from build123d import *

# Parameters (mm, degrees)
SKETCH2_W           = 1200
SKETCH2_H           = 1200
BOSS_EXTRUDE1_DEPTH = 600
SHELL1_T            = -100
SKETCH4_W           = 1200
SKETCH4_H           = 1200
BOSS_EXTRUDE2_DEPTH = 100
SKETCH5_R           = 129.5
CUT_EXTRUDE2_DEPTH  = 601
SKETCH7_W           = 130
SKETCH7_H           = 130
CUT_EXTRUDE3_DEPTH  = 146
CIRPATTERN1_COUNT   = 4
SKETCH8_R           = 120
CUT_EXTRUDE4_DEPTH  = 100


with BuildPart() as part:
    # Sketch2 → Boss-Extrude1 (new body)
    with BuildSketch(Plane.XY):
        Rectangle(SKETCH2_W, SKETCH2_H)
    extrude(amount=BOSS_EXTRUDE1_DEPTH)

    # Shell1
    shell1_openings = [part.faces().sort_by_distance(p)[0] for p in [
        (0, 0, 600),
    ]]
    offset(amount=SHELL1_T, openings=shell1_openings, kind=Kind.INTERSECTION)

    # Sketch4 → Boss-Extrude2 (add)
    with BuildSketch(Plane.XY.offset(600)):
        Rectangle(SKETCH4_W, SKETCH4_H)
    extrude(amount=-BOSS_EXTRUDE2_DEPTH)

    # Sketch5 → Cut-Extrude2 (cut, through all)
    with BuildSketch(Plane(origin=(0, 0, 0), x_dir=(-1, 0, 0), z_dir=(0, 0, -1))):
        Circle(SKETCH5_R)
    extrude(amount=-CUT_EXTRUDE2_DEPTH, mode=Mode.SUBTRACT)

    # Sketch7 → Cut-Extrude3 (cut)
    with BuildSketch(Plane(origin=(0, 0, 0), x_dir=(-1, 0, 0), z_dir=(0, 0, -1))):
        with Locations((0, 310)):
            Rectangle(SKETCH7_W, SKETCH7_H)
    cut_extrude3 = extrude(amount=-CUT_EXTRUDE3_DEPTH, mode=Mode.SUBTRACT)

    # CirPattern1: Cut-Extrude3 ×4 about axis
    cirpattern1_axis = Axis((0, 0, 0), (0, 0, 1))
    for i in range(1, CIRPATTERN1_COUNT):
        add(cut_extrude3.rotate(cirpattern1_axis, i * 360 / CIRPATTERN1_COUNT), mode=Mode.SUBTRACT)

    # Sketch8 → Cut-Extrude4 (cut)
    with BuildSketch(Plane.XZ.offset(600)):
        with Locations((-344.367385343, 324.291039311)):
            Circle(SKETCH8_R)
    extrude(amount=-CUT_EXTRUDE4_DEPTH, mode=Mode.SUBTRACT)


solid = part.part
Input: part model. Units: mm. Frame: model coordinates. A direction names the side the tool comes from. Coordinates: 2 decimals unless noted, no trailing zeros. Loops run counter-clockwise (first coordinate to the right, second up) from the corner with the lowest first, then second, coordinate; pieces in that order, holes last. Notation, with made-up numbers: (-24, -20) - (-17, -20) arc R17 cw to (-17, 9) - close; hole circle Ø10 at (15.25, 48.5). An arc over 180 degrees is marked (long way). Answer in a Markdown table with one row per item. Add a question column.
Item 1: Section query B-B on x = -481.5. Return the cut outline in (y, z).
Item 2: Access query for faces 4 (the cylindrical face through (-279.86, -550.7, 425.48)), 5 (the flat face through (-1, -245, 49)), 6 (the flat face through (-7, 500, 297)). Directions: +Z, -Z, +X, -X, +Y, -Y. A direction counts if a zero-diameter tool reaches every point of the face in a straight line with its end or side. Return the directions, or none.
Item 3: Contact query for a flat-ended pin moving along its axis: P1, Ø10, axis at x = -28, y = -214, coming from the -Z side. Output: stop coordinate, or through.
Item 4: Section query A-A on y = 0. Return the cut outline in (x, z), then the cut area to 3 significant figures.
Item 5: Line query: line 1 along Z through (x, y) = (475.5, 194.5); line 2 along X through (y, z) = (252, 200). Output: solid intervals per line, ascending. Write a range as [from, to].
Item 6: Mould query, pull axis X, two halves, no side actions, for faces 1 (the flat face through (-600, -8, 296)), 2 (the flat face through (-8, 142, 600)), 3 (the flat face through (-309, 65, 49)). Classes: released by +X, released by -X, zero draft, split by the parting line, or undercut.
Recorded:
| question | item | result |
|---|---|---|
| 1 | outline | (-600, 0) - (600, 0) - (600, 600) - (-600, 600) - close; hole (-500, 100) - (500, 100) - (500, 500) - (-500, 500) - close |
| 2 | face 4 | -Y |
| 2 | face 5 | -Z |
| 2 | face 6 | none |
| 3 | P1 | z = 0 |
| 4 | outline | (-600, 0) - (-375, 0) - (-375, 100) - (-500, 100) - (-500, 500) - (-129.5, 500) - (-129.5, 600) - (-600, 600) - close; (-245, 0) - (-129.5, 0) - (-129.5, 100) - (-245, 100) - close; (129.5, 0) - (245, 0) - (245, 100) - (129.5, 100) - close; (129.5, 500) - (500, 500) - (500, 100) - (375, 100) - (375, 0) - (600, 0) - (600, 600) - (129.5, 600) - close |
| 4 | area | 242,000 mm^2 |
| 5 | line 1 | [0, 100], [500, 600] |
| 5 | line 2 | [-600, -500], [500, 600] |
| 6 | face 1 | released by -X |
| 6 | face 2 | zero draft |
| 6 | face 3 | undercut |
